The model under review builds one solid part; all positions refer to its coordinate system, in mm. A direction names the side the tool comes from. Round coordinates to 2 decimals unless told otherwise and drop trailing zeros. Order: outer loops, then holes, each group sorted by start corner. A loop starts at its lowest first (then second) coordinate and runs counter-clockwise, first axis right, second up. Notation, with made-up numbers: (-34.5, 17) - (12.5, 17) arc R5 ccw to (12.5, 25) - close; hole circle Ø11 at (-4, -24). An arc over 180 degrees is marked (long way). One line per question, with ' | ' between items. Start each with the question number.
Item 1: Add section B-B on y = 44. State the section outline as (x, z) points, and give its area (3 significant figures).
Item 2: Add section A-A on z = -13.5. State the section outline as (x, y) points.
Item 3: Tool access review of faces 1 (the face through (-200, 35, 2)), 2 (the face through (197.535, 37.932, -12.459)), 3 (the face through (-192.15, 30.42, 141.99)): name each direction out of +Z, -Z, +X, -X, +Y, -Y from which nothing blocks a thin tool from reaching the whole face with its end or side.
Item 4: Draft analysis for pull direction Z (two halves, no side actions). For faces 4 (the face through (-3, 70, -2)), 5 (the face through (-3, 35, 150)), 6 (the face through (-192.15, 30.42, -141.99)), state which applies: +Z half, -Z half, draft (parallel to the pull), parting line (faces both ways), or undercut.
Item 5: Insertion check: pin 1 Ø6 at (x, z) = (-16, 42) entering from -Y. The pin has a flat end and moves straight along its axis. Give the tip position at first contact, or say it passes through.
Item 6: For L1, parallel to Y at x = -110, z = -146; L2, parallel to Z at x = 155, y = 10; L3, parallel to Y at x = 197.6, z = 13.5, list the stretches that pass through material, from the lowest coordinate up. Write a range as [from, to].
Item 7: Add section C-C on x = 74.5. State the section outline as (y, z) points.
from build123d import *

# Parameters (mm, degrees)
SKETCH1_W           = 400
SKETCH1_H           = 300
BOSS_EXTRUDE1_DEPTH = 70
SKETCH2_W           = 390
SKETCH2_H           = 290
CUT_EXTRUDE1_DEPTH  = 60
FILLET2_R           = 10
SKETCH6_R           = 8
CUT_EXTRUDE3_DEPTH  = 10
SKETCH7_R           = 3.535
CUT_EXTRUDE4_DEPTH  = 459


with BuildPart() as part:
    # Sketch1 → Boss-Extrude1 (new body)
    with BuildSketch(Plane(origin=(0, 0, 0), x_dir=(1, 0, 0), z_dir=(0, 1, 0))):
        Rectangle(SKETCH1_W, SKETCH1_H)
    extrude(amount=BOSS_EXTRUDE1_DEPTH)

    # Sketch2 → Cut-Extrude1 (cut)
    with BuildSketch(Plane.XZ):
        Rectangle(SKETCH2_W, SKETCH2_H)
    extrude(amount=-CUT_EXTRUDE1_DEPTH, mode=Mode.SUBTRACT)

    # Fillet2
    fillet2_edges = [part.edges().sort_by_distance(p)[0] for p in [
        (195, 30, 145),
        (195, 30, -145),
        (-195, 30, -145),
        (-195, 30, 145),
    ]]
    fillet(fillet2_edges, radius=FILLET2_R)

    # Sketch6 → Cut-Extrude3 (cut)
    with BuildSketch(Plane(origin=(200, 0, 0), x_dir=(0, 0, -1), z_dir=(1, 0, 0))):
        with Locations((-13.5, 30)):
            Circle(SKETCH6_R)
        with Locations((13.5, 30)):
            Circle(SKETCH6_R)
    extrude(amount=-CUT_EXTRUDE3_DEPTH, mode=Mode.SUBTRACT)

    # Sketch7 → Cut-Extrude4 (cut)
    with BuildSketch(Plane.XY.offset(150)):
        with Locations((-110, 17.670088152)):
            Circle(SKETCH7_R)
        with Locations((110, 17.670088152)):
            Circle(SKETCH7_R)
    extrude(amount=-CUT_EXTRUDE4_DEPTH, mode=Mode.SUBTRACT)


solid = part.part
Determined:
1) outline: (-200, -150) - (200, -150) - (200, 150) - (-200, 150) - close; hole (-195, -135) arc R10 ccw to (-185, -145) - (185, -145) arc R10 ccw to (195, -135) - (195, 135) arc R10 ccw to (185, 145) - (-185, 145) arc R10 ccw to (-195, 135) - close | area: 6,990 mm2
2) outline: (-200, 0) - (-195, 0) - (-195, 60) - (195, 60) - (195, 38) - (200, 38) - (200, 70) - (-200, 70) - close; (195, 0) - (200, 0) - (200, 22) - (195, 22) - close
3) face 1: +Z, -Z, -X, +Y, -Y | face 2: +X | face 3: -Y
4) face 4: draft | face 5: +Z half | face 6: undercut
5) pin 1: y = 60
6) L1: [0, 14.14], [21.21, 70] | L2: [-150, -145], [145, 150] | L3: [0, 22], [38, 70]
7) outline: (0, -150) - (70, -150) - (70, 150) - (0, 150) - (0, 145) - (60, 145) - (60, -145) - (0, -145) - close
